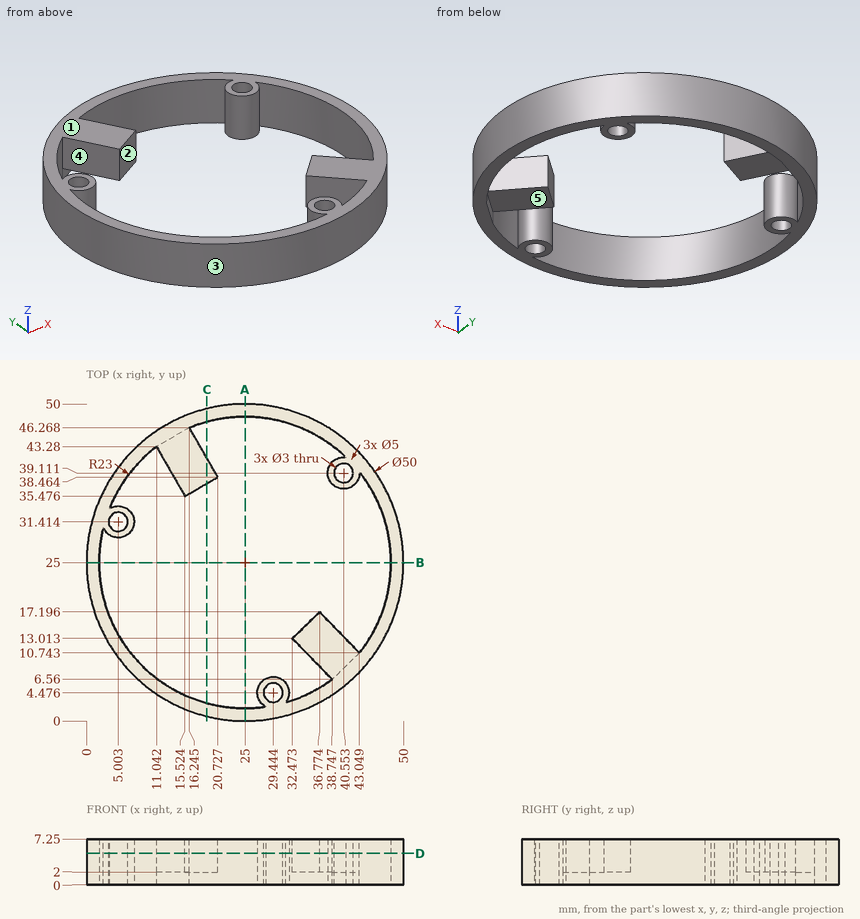
Can you work these out from the drawing? Everything is in mm from the part's minimum corner. A direction names the side the tool comes from. Round coordinates to 2 decimals unless told otherwise and drop trailing zeros. Loops run counter-clockwise (first coordinate to the right, second up) from the corner with the lowest first, then second, coordinate; pieces in that order, holes last. Notation, with made-up numbers: (41.25, 84.25) - (73.25, 84.25) arc R8 cw to (73.25, 95.25) - close; hole circle Ø11 at (-26.5, -28.75). An arc over 180 degrees is marked (long way). One line per question, with ' | ' between items. Start each with the question number.
Q1. Please list where these lines run through material, in increasing order: line 1 (Y direction, x = 5.5, z = 1.75) (1 decimal); line 2 (X direction, y = 38, z = 0.5) (1 decimal); line 3 (Y direction, x = 25, z = 5.5). Write a range as [from, to].
Q2. I want a section at A-A (x = 25). Write out the boundary of the cut face in (y, z).
Q3. I want a section at C-C (x = 19). Write out the boundary of the cut face in (y, z).
Q4. I want a section at D-D (z = 5). Write out the boundary of the cut face in (x, y) (1 decimal).
Q5. For the marked faces 4 and 5, which set-ups out of +Z, -Z, +X, -X, +Y, -Y let a thin tool reach every point of the face, with its end or its side?
Q6. We'd pull the mould along X, two halves only. Please class the marked faces 1, 2 and 3: +X half, -X half, draft (parallel to the pull), parting line (faces both ways), or undercut.
Q7. Will these pins go through, and if not, where does the flat tip stop? pin 1 (4 mm diameter, centred on y = 16, z = 1, fed in from +X); pin 2 (3.5 mm diameter, centred on x = 40.55, y = 39.11, fed in from +Z); pin 3 (4 mm diameter, centred on y = 8, z = 3, fed in from +X); pin 4 (10.5 mm diameter, centred on x = 16.5, y = 40, fed in from -Z).
Response values:
1) line 1: y = [9.4, 12.8], [29, 30], [32.8, 33.9], [37.2, 40.6] | line 2: x = [3.6, 6], [38.3, 39.5], [41.6, 42.8], [44, 46.4] | line 3: y = [0, 2], [48, 50]
2) outline: (0, 0) - (2, 0) - (2, 7.25) - (0, 7.25) - close; (48, 0) - (50, 0) - (50, 7.25) - (48, 7.25) - close
3) outline: (0.73, 0) - (2.8, 0) - (2.8, 7.25) - (0.73, 7.25) - close; (37.47, 2) - (41.47, 2) - (41.47, 7.25) - (37.47, 7.25) - close; (47.2, 0) - (49.27, 0) - (49.27, 7.25) - (47.2, 7.25) - close
4) outline: circle Ø50 at (25, 25); hole (2.7, 30.5) arc R23 ccw to (28.3, 2.2) arc R2.5 cw (long way) to (31.4, 2.9) arc R23 ccw to (38.7, 6.6) - (32.5, 13) - (36.8, 17.2) - (43, 10.7) arc R23 ccw to (43, 39.3) arc R2.5 cw (long way) to (40.9, 41.6) arc R23 ccw to (16.2, 46.3) - (20.7, 38.5) - (15.5, 35.5) - (11, 43.3) arc R23 ccw to (3.6, 33.5) arc R2.5 cw (long way) to start; hole circle Ø3 at (5, 31.4); hole circle Ø3 at (29.4, 4.5); hole circle Ø3 at (40.6, 39.1)
5) face 4: +Z, -Z | face 5: -Z
6) face 1: draft | face 2: undercut | face 3: parting line
7) pin 1: stops at x = 49 | pin 2: stops at z = 7.25 | pin 3: stops at x = 45 | pin 4: stops at z = 2
